Autodesk Inventor part; units mm, degrees
ref_plane "YZ Plane" through (0, 0, 0) normal (1, 0, 0) x (0, 1, 0)
ref_plane "XZ Plane" through (0, 0, 0) normal (0, 1, 0) x (-1, 0, 0)
ref_plane "XY Plane" through (0, 0, 0) normal (0, 0, 1) x (1, 0, 0)
sketch "master" plane through (0, 0, 0) normal (0, 0, 1) x (1, 0, 0)
  line L0 (-8.5, -8.5) -> (8.5, -8.5)
  line L1 (8.5, -8.5) -> (8.5, 8.5)
  line L2 (8.5, 8.5) -> (-8.5, 8.5)
  line L3 (-8.5, 8.5) -> (-8.5, -8.5)
  line L4 (-8.5, -8.5) -> (8.5, 8.5) construction
  line L5 (8.5, -8.5) -> (-8.5, 8.5) construction
  circle A0 centre (-0.65, 0) radius 5.65
  line L6 (5, 0) -> (8.5, 0) construction
  point P0 (0, 0)
  point P1 (0, 0)
  dimension "d1" = 11.3
  dimension "d0" = 17
  dimension "d12" = 3.5
  dimension "d14" = 9.15
  dimension "d22" = 0.65
extrude "body" add sketch "master" against normal blind 3.5 contours L3 L2 L1 L0 | A0
sketch "Sketch2" plane through (-8.5, -8.5, 0) normal (-1, 0, 0) x (0, 0, 1)
  line L0 (0, 17) -> (0, 0)
  line L1 (0, 17) -> (-3.5, 17)
  line L2 (-3.5, 0) -> (-3.5, 17)
  line L3 (0, 0) -> (-3.5, 0)
  line L4 (0, 17) -> (0, 0)
  line L5 (-3, 16.16) -> (-0.25, 16.16)
  line L6 (-0.25, 16.16) -> (-0.25, 5.4)
  line L7 (-0.25, 5.4) -> (-3, 5.4)
  line L8 (-3, 5.4) -> (-3, 16.16)
  point P0 (0, 8.5)
  dimension "d4" = 5.4
  dimension "d5" = 0.84
  dimension "d6" = 0.25
  dimension "d7" = 0.5
extrude "outlet" cut sketch "Sketch2" against normal blind 15 contours L5 L6 L7 L8
extrude "Extrusion3" cut sketch "master" against normal up to surface (3 mm away) contours A0
sketch "Sketch3" plane through (-8.5, -8.5, 0) normal (0, -1, 0) x (1, 0, 0)
  line L0 (17, 0) -> (17, -3.5)
  arc A0 (17, -1.75) -> (17.6, -1.15) centre (17, -1.15) ccw
  line L1 (17.6, -1.15) -> (17.6, 1)
  point P0 (8.5, 0)
  dimension "d15" = 1
  dimension "d16" = 0.6
sketch "Sketch4" plane through (8.5, -8.5, 0) normal (1, 0, 0) x (0, 0, -1)
  line L0 (1.35, 2) -> (1.35, 0)
  line L1 (1.35, 0) -> (1.75, 0)
  line L2 (1.75, 0) -> (1.75, 2)
  line L3 (1.75, 2) -> (1.35, 2)
  line L4 (1.35, 2) -> (1.75, 0) construction
  line L5 (1.35, 0) -> (1.75, 2) construction
  line L6 (0, 0) -> (3.5, 0)
  point P0 (0, 8.5)
  point P1 (1.55, 1)
  dimension "d17" = 2
  dimension "d18" = 0.4
sweep "Sweep1" add profiles "Sketch4" path "Sketch3" path curves A0 L1
fillet "Fillet1" radius 0.2 5 edges at (8.5, -8.5, -2.625) (8.5, 8.5, -1.75) (-8.5, -8.5, -1.75) (-8.5, 8.5, -1.75) (8.5, -8.5, -0.675)
properties part number "fan_sunon_ub3h3_500" material "PC/ABS Plastic"
Here's how the part is built. I have some questions about the finished solid (model axes, mm). A direction names the side the tool comes from. Coordinates: 2 decimals unless noted, no trailing zeros. Order: outer loops, then holes, each group sorted by start corner. A loop starts at its lowest first (then second) coordinate and runs counter-clockwise, first axis right, second up.
1) We'd pull the mould along Y, two halves only. Please class faces 5 (the face through (-1, 7.66, -2)), 6 (the face through (4, 4, 0)), 7 (the face through (0, -8.5, -2)), 8 (the face through (0, 8.5, -2)): +Y half, -Y half, draft (parallel to the pull), parting line (faces both ways), or undercut.
2) I need wall thicknesses on line 1 (Y direction, x = -5.75, z = -2.5); line 2 (Y direction, x = -0.65, z = -1.8); line 3 (Z direction, x = 5, y = 4.5). Which ranges of each line are inside material? Lowest first, please.
3) Which directions (+Z, -Z, +X, -X, +Y, -Y) give clear straight access to the entire face, cutting with the end or side of a thin tool? Please do faces 1 (the face through (8.7, -7, 0)), 2 (the face through (-8.5, -4, -2)), 3 (the face through (-1.875, -5.516, -1.146)), 4 (the face through (-1, 6, -0.25)).
4) Imagine slicing it at B-B on z = -2.7. List the corners of the cut face in (x, y) for me, and give its area (3 significant figures).
5) Imagine slicing it at D-D on y = 7. List the corners of the cut face in (x, z) for me, and give its area (4 significant figures).
6) Will these pins go through, and if not, where does the flat tip stop? pin 1 (5 mm diameter, centred on x = 0.5, y = 2, fed in from +Z); pin 2 (2 mm diameter, centred on x = 4.5, y = 0.5, fed in from +Z); pin 3 (1.4 mm diameter, centred on y = 5, z = -1.5, fed in from -X).
7) Imagine slicing it at C-C on x = 6.25. List the corners of the cut face in (y, z) for me, and give its area (3 significant figures).
8) Imagine slicing it at A-A on y = 0.75. List the corners of the cut face in (x, z) for me, and give its area (4 significant figures).
Response values:
1. face 5: undercut
1. face 6: draft
1. face 7: -Y half
1. face 8: +Y half
2. line 1: y = -8.5 to -3.1, 7.66 to 8.5
2. line 2: y = -8.5 to -5.65, 7.66 to 8.5
2. line 3: z = -3.5 to -3, -0.25 to 0
3. face 1: +Z, +Y, -Y
3. face 2: +Z, -Z, -X, +Y, -Y
3. face 3: +Z
3. face 4: -X
4. outline: (-8.5, -8.3) arc R0.2 ccw to (-8.3, -8.5) - (8.3, -8.5) arc R0.2 ccw to (8.5, -8.3) - (8.5, 8.3) arc R0.2 ccw to (8.3, 8.5) - (-8.3, 8.5) arc R0.2 ccw to (-8.5, 8.3) - (-8.5, 7.66) - (6.5, 7.66) - (6.5, -3.1) - (4.07, -3.1) arc R5.65 cw to (-5.37, -3.1) - (-8.5, -3.1) - close
4. area: 111 mm2
5. outline: (-8.5, -3.5) - (8.5, -3.5) - (8.5, 0) - (-8.5, 0) - (-8.5, -0.25) - (6.5, -0.25) - (6.5, -3) - (-8.5, -3) - close
5. area: 18.25 mm2
6. pin 1: stops at z = -3
6. pin 2: stops at z = 0
6. pin 3: stops at x = 6.5
7. outline: (-8.5, -3.5) - (8.5, -3.5) - (8.5, 0) - (-8.5, 0) - close; hole (-3.1, -3) - (7.66, -3) - (7.66, -0.25) - (-3.1, -0.25) - close
7. area: 29.9 mm2
8. outline: (-8.5, -3.5) - (8.5, -3.5) - (8.5, 0) - (4.95, 0) - (4.95, -0.25) - (6.5, -0.25) - (6.5, -3) - (-8.5, -3) - close; (-8.5, -0.25) - (-6.25, -0.25) - (-6.25, 0) - (-8.5, 0) - close
8. area: 15.45 mm2
